Part model, mm, in its own coordinate system. A direction names the side the tool comes from. Round coordinates to 2 decimals unless told otherwise and drop trailing zeros. Loops run counter-clockwise (first coordinate to the right, second up) from the corner with the lowest first, then second, coordinate; pieces in that order, holes last.
(1) Cut at A-A on z = 30.75. List the corners of the cut face in (x, y).
(2) Mould opens along Z. For faces 1 (the face through (-24, 4, 32)), 2 (the face through (-23.51, 1.97, 40.05)), 3 (the face through (-24, -9, 17.625)), 4 (the face through (-40.1, 1.972, 44.774)) say: +Z half, -Z half, draft (parallel to the pull), parting line (faces both ways), or undercut.
(3) Tool access for faces 5 (the face through (-24, 2, 47.625)), 6 (the face through (-24.018, -10.846, 27.625)): list every direction of +Z, -Z, +X, -X, +Y, -Y with a clear straight run to the whole face (end or side of a thin tool).
(4) Cut at C-C on x = -10. List the corners of the cut face in (y, z), then the cut area to 3 significant figures.
(5) Probe probe 1 along Y at (x, z) = (-22.5, 30); probe 2 along Z at (x, y) = (-30, -1.5); probe 3 along Z at (x, y) = (-11, -4.5). List the from-to ranges inside material, lowest first.
(6) Flat gauge pins, fed straight in: pin 1 (8.5 mm diameter, centred on x = -16, z = 35, fed in from -Y); pin 2 (1.6 mm diameter, centred on x = -24.11, z = 40.13, fed in from +Y). Where does each tip first touch, or does it go through?
(7) Cut at D-D on z = 24.5. List the corners of the cut face in (x, y).
(8) Cut at B-B on y = -20. List the corners of the cut face in (x, z), then the cut area to 3 significant figures.
from build123d import *

# Parameters (mm, degrees)
CROQUIS2_R              = 0.6
SALIENTE_EXTRUIR1_DEPTH = 4
SALIENTE_EXTRUIR2_DEPTH = 22
REDONDEO1_R             = 10
REDONDEO2_R             = 10


with BuildPart() as part:
    # Croquis2 → Saliente-Extruir1 (new body)
    with BuildSketch(Plane(origin=(0, 0, 0), x_dir=(1, 0, 0), z_dir=(0, 1, 0))):
        with BuildLine():
            Line((-43.107082341, -17.625158928), (-5.107082341, -17.625158928))
            Line((-5.107082341, -17.625158928), (-5.107082341, -37.625158928))
            ThreePointArc((-5.107082341, -37.625158928), (-8.036014529, -44.69622674), (-15.107082341, -47.625158928))
            Line((-15.107082341, -47.625158928), (-33.107082341, -47.625158928))
            ThreePointArc((-33.107082341, -47.625158928), (-40.178150153, -44.69622674), (-43.107082341, -37.625158928))
            Line((-43.107082341, -37.625158928), (-43.107082341, -17.625158928))
        make_face()
        with Locations(Location((-24.107082341, -40.125158928, 0), (0, 0, 270))):
            Circle(CROQUIS2_R, mode=Mode.SUBTRACT)
    extrude(amount=SALIENTE_EXTRUIR1_DEPTH)

    # Croquis3 → Saliente-Extruir2 (add)
    with BuildSketch(Plane.XZ):
        with BuildLine():
            Line((-43.107082341, 17.625158928), (-5.107082341, 17.625158928))
            Line((-5.107082341, 17.625158928), (-5.107082341, 37.625158928))
            ThreePointArc((-5.107082341, 37.625158928), (-24.107082341, 27.625158928), (-43.107082341, 37.625158928))
            Line((-43.107082341, 37.625158928), (-43.107082341, 17.625158928))
        make_face()
    extrude(amount=SALIENTE_EXTRUIR2_DEPTH)

    # Redondeo1
    redondeo1_edges = [part.edges().sort_by_distance(p)[0] for p in [
        (-43.107082341, -11, 37.625158928),
    ]]
    fillet(redondeo1_edges, radius=REDONDEO1_R)

    # Redondeo2
    redondeo2_edges = [part.edges().sort_by_distance(p)[0] for p in [
        (-5.107082341, -11, 37.625158928),
    ]]
    fillet(redondeo2_edges, radius=REDONDEO2_R)


solid = part.part
Final values:
1. outline: (-43.11, 0) - (-5.11, 0) - (-5.11, 4) - (-43.11, 4) - close
2. face 1: draft
2. face 2: undercut
2. face 3: -Z half
2. face 4: +Z half
3. face 5: +Z, +X, -X, +Y, -Y
3. face 6: +Z, -Y
4. outline: (-22, 17.63) - (4, 17.63) - (4, 46.22) - (0, 46.22) - (0, 27.47) - (-22, 27.47) - close
4. area: 331 mm2
5. probe 1: y = 0 to 4
5. probe 2: z = 17.63 to 28.39
5. probe 3: z = 17.63 to 27.99
6. pin 1: stops at y = 0
6. pin 2: stops at y = 4
7. outline: (-43.11, 0) - (-41.37, 0) - (-41.37, -22) - (-6.84, -22) - (-6.84, 0) - (-5.11, 0) - (-5.11, 4) - (-43.11, 4) - close
8. outline: (-43.11, 17.63) - (-5.11, 17.63) - (-5.11, 18.87) arc R10 ccw to (-17.83, 28.5) arc R23.05 cw to (-30.38, 28.5) arc R10 ccw to (-43.11, 18.87) - close
8. area: 372 mm2
